Autodesk Inventor part; units mm, degrees
ref_plane "YZ Plane" through (0, 0, 0) normal (1, 0, 0) x (0, 1, 0)
ref_plane "XZ Plane" through (0, 0, 0) normal (0, 1, 0) x (-1, 0, 0)
ref_plane "XY Plane" through (0, 0, 0) normal (0, 0, 1) x (1, 0, 0)
sketch "Sketch1" plane through (0, 0, 0) normal (0, 0, 1) x (1, 0, 0)
  line L0 (0, 0) -> (20, 0)
  line L1 (20, 0) -> (20, -2.7984)
  line L2 (0, -2.7984) -> (0, 0)
  line L3 (0, 0) -> (20, 0)
  line L4 (20, 0) -> (20, -50)
  line L5 (20, -50) -> (0, -50)
  line L6 (0, -50) -> (0, 0)
  line L7 (0, 0) -> (5, 0)
  line L8 (0, -5) -> (0, 0)
  circle A0 centre (5, -5) radius 1.651
  line L9 (20, 0) -> (15, 0)
  line L10 (15, -5) -> (20, -5)
  line L11 (20, -5) -> (20, 0)
  circle A1 centre (15, -5) radius 1.651
  dimension "d1" = 20
  dimension "d2" = 50
  dimension "d6" = 5
  dimension "d7" = 5
  dimension "d9" = 3.302
extrude "Extrusion1" add sketch "Sketch1" along normal blind 5
sketch "Sketch2" plane through (0, 0, 5) normal (0, 0, 1) x (1, 0, 0)
  line L0 (20, 0) -> (0, 0)
  line L1 (10, 0) -> (5, 0)
  line L2 (5, 0) -> (5, 5)
  line L3 (5, 5) -> (10, 5)
  line L4 (10, 5) -> (10, 0)
  line L5 (10, 5) -> (2.5, 5)
  line L6 (2.5, 5) -> (2.5, 7.5)
  line L7 (2.5, 7.5) -> (10, 7.5)
  line L8 (10, 7.5) -> (10, 5)
  line L9 (2.5, 7.5) -> (17.5, 7.5)
  line L10 (17.5, 7.5) -> (17.5, 5)
  line L11 (17.5, 5) -> (2.5, 5)
  line L12 (2.5, 5) -> (2.5, 7.5)
  line L13 (10, 5) -> (15, 5)
  line L14 (15, 5) -> (15, 0)
  line L15 (15, 0) -> (10, 0)
  line L16 (10, 0) -> (10, 5)
  dimension "d12" = 5
  dimension "d13" = 5
  dimension "d14" = 7.5
  dimension "d15" = 2.5
  dimension "d16" = 15
  dimension "d17" = 2.5
  dimension "d18" = 5
  dimension "d19" = 5
extrude "Extrusion2" add sketch "Sketch2" against normal blind 5
sketch "Sketch3" plane through (0, 0, 0) normal (0, 0, -1) x (-1, 0, 0)
  line L0 (-5, 0) -> (-5, 5)
  line L1 (-5, 0) -> (-15, 0)
  line L2 (-15, 0) -> (-15, 5)
  line L3 (-15, 5) -> (-5, 5)
  line L4 (-5, 5) -> (-5, 0)
  point P0 (0, 0)
extrude "Extrusion3" cut sketch "Sketch3" against normal blind 1
sketch "Sketch4" plane through (0, 0, 0) normal (0, 0, -1) x (-1, 0, 0)
  line L0 (-5, 0) -> (0, 0)
  line L1 (-20, -50) -> (0, -50)
  line L2 (0, 0) -> (-20, 0)
  line L3 (-20, 0) -> (-20, -50)
  line L4 (-20, -50) -> (0, -50)
  line L5 (0, -50) -> (0, 0)
  line L6 (0, -50) -> (-5, -50)
  line L7 (-5, -50) -> (-5, -30)
  line L8 (-5, -30) -> (0, -30)
  line L9 (0, -30) -> (0, -50)
  line L10 (0, -50) -> (0, 0)
  line L11 (0, -50) -> (-5, -50)
  line L12 (-5, -50) -> (-5, -30)
  line L13 (-5, -30) -> (0, -30)
  line L14 (0, -30) -> (0, -50)
  line L15 (0, -50) -> (-20, -50)
  line L16 (-20, -50) -> (-20, -45)
  line L17 (-20, -45) -> (0, -45)
  line L18 (0, -45) -> (0, -50)
  dimension "d28" = 5
  dimension "d29" = 20
  dimension "d30" = 5
  dimension "d31" = 20
  dimension "d32" = 20
  dimension "d33" = 5
extrude "Extrusion4" add sketch "Sketch4" along normal blind 15 contours L17 L7 L1 L3 | L5 L1 L7 L17
sketch "Sketch5" plane through (0, 0, 5) normal (0, 0, 1) x (1, 0, 0)
  line L0 (20, -50) -> (20, 0)
  line L1 (20, 0) -> (0, 0)
  line L2 (0, 0) -> (0, -50)
  line L3 (0, -50) -> (20, -50)
  line L4 (20, -50) -> (20, 0)
  line L5 (10, -50) -> (15, -50)
  line L6 (15, -50) -> (15, -55)
  line L7 (15, -55) -> (10, -55)
  line L8 (10, -55) -> (10, -50)
  line L9 (15, -55) -> (5, -55)
  line L10 (5, -55) -> (5, -50)
  line L11 (5, -50) -> (15, -50)
  line L12 (15, -50) -> (15, -55)
  line L13 (10, -55) -> (17.5, -55)
  line L14 (17.5, -55) -> (17.5, -57.5)
  line L15 (17.5, -57.5) -> (10, -57.5)
  line L16 (10, -57.5) -> (10, -55)
  line L17 (17.5, -57.5) -> (2.5, -57.5)
  line L18 (2.5, -57.5) -> (2.5, -55)
  line L19 (2.5, -55) -> (17.5, -55)
  line L20 (17.5, -55) -> (17.5, -57.5)
  dimension "d36" = 5
  dimension "d37" = 5
  dimension "d38" = 10
  dimension "d39" = 5
  dimension "d40" = 7.5
  dimension "d41" = 2.5
  dimension "d42" = 15
  dimension "d43" = 2.5
extrude "Extrusion5" add sketch "Sketch5" against normal blind 5 contours L6 L7 L8 L3 | L8 L9 L10 L3 | L13 L14 L15 L16 L7 | L16 L17 L18 L19 L9
sketch "Sketch6" plane through (0, 0, 0) normal (0, 0, -1) x (-1, 0, 0)
  line L0 (-5, -55) -> (-5, -50)
  line L1 (-15, -50) -> (-5, -50)
  line L2 (-5, -55) -> (-15, -55)
  line L3 (-15, -55) -> (-15, -50)
  line L4 (-15, -50) -> (-5, -50)
  line L5 (-5, -50) -> (-5, -55)
  point P0 (0, 0)
extrude "Extrusion6" cut sketch "Sketch6" against normal blind 1
sketch "Sketch8" plane through (0, -45, 0) normal (0, 1, 0) x (1, 0, 0)
  line L0 (0, 15) -> (20, 15)
  line L1 (0, 15) -> (20, 15)
  line L2 (20, 15) -> (20, 0)
  line L3 (20, 0) -> (0, 0)
  line L4 (0, 0) -> (0, 15)
  line L5 (0, 0) -> (0, 15)
  line L6 (0, 7.5) -> (20, 7.5)
  line L7 (20, 0) -> (20, 15)
  line L8 (20, 0) -> (0, 15)
  line L9 (20, 15) -> (0, 0)
  line L10 (10, 7.5) -> (10, 15)
  line L11 (10, 7.5) -> (10, 0)
  line L12 (10, 7.5) -> (0, 0)
  line L13 (10, 7.5) -> (20, 0)
  line L14 (10, 7.5) -> (0, 15)
  line L15 (10, 7.5) -> (20, 15)
  circle A0 centre (5, 3.75) radius 1.651
  circle A1 centre (15, 3.75) radius 1.651
  circle A2 centre (15, 11.25) radius 1.651
  circle A3 centre (5, 11.25) radius 1.651
  dimension "d48" = 3.302
  dimension "d49" = 3.302
  dimension "d50" = 3.302
  dimension "d51" = 3.302
extrude "Extrusion7" cut sketch "Sketch8" against normal blind 5 contours A3 L8 | L8 A3 | A2 L9 | L9 A2 | A1 L8 | L8 A1 | A0 L9 | L9 A0
sketch "Sketch9" plane through (2.5, -57.5, 5) normal (0, -1, 0) x (1, 0, 0)
  line L0 (15, 0) -> (0, 0)
  line L1 (7.5, 0) -> (8, 0)
  line L2 (8, 0) -> (8, -0.5)
  line L3 (8, -0.5) -> (7.5, -0.5)
  line L4 (7.5, -0.5) -> (7.5, 0)
  line L5 (7.5, 0) -> (7, 0)
  line L6 (7, 0) -> (7, -0.5)
  line L7 (7, -0.5) -> (7.5, -0.5)
  line L8 (7.5, -0.5) -> (7.5, 0)
  point P0 (-2.5, -5)
  dimension "d54" = 0.5
  dimension "d55" = 0.5
  dimension "d56" = 0.5
  dimension "d57" = 0.5
extrude "Extrusion8" cut sketch "Sketch9" against normal blind 500
sketch "Sketch10" plane through (0, -45, 0) normal (0, 1, 0) x (1, 0, 0)
  circle A0 centre (5, 11.25) radius 1.651
  circle A1 centre (5, 11.25) radius 1.651
  circle A2 centre (5, 3.75) radius 1.651
  circle A3 centre (5, 3.75) radius 1.651
  circle A4 centre (15, 11.25) radius 1.651
  circle A5 centre (15, 11.25) radius 1.651
  circle A6 centre (15, 3.75) radius 1.651
  circle A7 centre (15, 3.75) radius 1.651
  circle A8 centre (5, 11.25) radius 3
  circle A9 centre (15, 11.25) radius 3
  circle A10 centre (5, 3.75) radius 3
  circle A11 centre (15, 3.75) radius 3
  line L0 (5, 14.25) -> (7.5981, 12.75)
  line L1 (7.5981, 12.75) -> (7.5981, 9.75)
  line L2 (7.5981, 9.75) -> (5, 8.25)
  line L3 (5, 8.25) -> (2.4019, 9.75)
  line L4 (2.4019, 9.75) -> (2.4019, 12.75)
  line L5 (2.4019, 12.75) -> (5, 14.25)
  line L6 (15, 14.25) -> (17.5981, 12.75)
  line L7 (17.5981, 12.75) -> (17.5981, 9.75)
  line L8 (17.5981, 9.75) -> (15, 8.25)
  line L9 (15, 8.25) -> (12.4019, 9.75)
  line L10 (12.4019, 9.75) -> (12.4019, 12.75)
  line L11 (12.4019, 12.75) -> (15, 14.25)
  line L12 (5, 6.75) -> (7.5981, 5.25)
  line L13 (7.5981, 5.25) -> (7.5981, 2.25)
  line L14 (7.5981, 2.25) -> (5, 0.75)
  line L15 (5, 0.75) -> (2.4019, 2.25)
  line L16 (2.4019, 2.25) -> (2.4019, 5.25)
  line L17 (2.4019, 5.25) -> (5, 6.75)
  line L18 (15, 6.75) -> (17.5981, 5.25)
  line L19 (17.5981, 5.25) -> (17.5981, 2.25)
  line L20 (17.5981, 2.25) -> (15, 0.75)
  line L21 (15, 0.75) -> (12.4019, 2.25)
  line L22 (12.4019, 2.25) -> (12.4019, 5.25)
  line L23 (12.4019, 5.25) -> (15, 6.75)
  point P0 (0, 0)
  dimension "d60" = 6
  dimension "d61" = 6
  dimension "d62" = 6
  dimension "d63" = 6
extrude "Extrusion9" cut sketch "Sketch10" against normal blind 2 contours L1 L2 L3 L4 L5 L0 | L7 L8 L9 L10 L11 L6 | L13 L14 L15 L16 L17 L12 | L19 L20 L21 L22 L23 L18
sketch "Sketch11" plane through (0, 0, 5) normal (0, 0, 1) x (1, 0, 0)
  circle A0 centre (5, -5) radius 1.651
  circle A1 centre (5, -5) radius 3
  circle A2 centre (15, -5) radius 1.651
  circle A3 centre (15, -5) radius 3
  line L0 (5, -2) -> (7.5981, -3.5)
  line L1 (7.5981, -3.5) -> (7.5981, -6.5)
  line L2 (7.5981, -6.5) -> (5, -8)
  line L3 (5, -8) -> (2.4019, -6.5)
  line L4 (2.4019, -6.5) -> (2.4019, -3.5)
  line L5 (2.4019, -3.5) -> (5, -2)
  line L6 (15, -2) -> (17.5981, -3.5)
  line L7 (17.5981, -3.5) -> (17.5981, -6.5)
  line L8 (17.5981, -6.5) -> (15, -8)
  line L9 (15, -8) -> (12.4019, -6.5)
  line L10 (12.4019, -6.5) -> (12.4019, -3.5)
  line L11 (12.4019, -3.5) -> (15, -2)
  point P0 (0, 0)
  dimension "d66" = 6
  dimension "d67" = 6
extrude "Extrusion10" cut sketch "Sketch11" against normal blind 2 contours L1 L2 L3 L4 L5 L0 | L7 L8 L9 L10 L11 L6
properties part number "Attachment"
The model under review builds one solid part; all positions refer to its coordinate system, in mm. A direction names the side the tool comes from. Round coordinates to 2 decimals unless told otherwise and drop trailing zeros. Write each loop counter-clockwise with the first axis right and the second up, starting at its lowest first coordinate (ties: lowest second). Pieces come first, ordered by that corner, then holes.
(1) We need section C-C on y = -21. Give the boundary of the cut face in (x, z), and give its area (3 significant figures).
(2) Insertion check: pin 1 (1.5 mm diameter, centred on y = -12, z = -1, fed in from -X); pin 2 (4 mm diameter, centred on x = 15, y = -4.5, fed in from +Z); pin 3 (5.5 mm diameter, centred on x = 4.5, z = -3.5, fed in from +Y); pin 4 (2 mm diameter, centred on x = 11, y = -8.5, fed in from -Z). Each pin has a flat end and moves straight along its axis. Give the tip position at first contact, or say it passes through.
(3) Machinability: for faces 4 (the flat face through (11.8, 5, 0.3)), 5 (the flat face through (16.3, -46, -13.5)), 6 (the flat face through (16.32, -7.24, 4.01)), 7 (the flat face through (10, 6, 0)), 8 (the flat face through (10, -56, 0)), which of the approach directions +Z, -Z, +X, -X, +Y, -Y give a long, thin tool a straight path to every point of the face, cutting with its end or side? Answer none if there is none.
(4) Wall thickness on L1, parallel to Z at x = 5, y = -48.5; L2, parallel to X at y = -49, z = -3.75; L3, parallel to Z at x = 6.5, y = -47.5: over which ranges is each line inside the solid? List them lowest first.
(5) We need section A-A on y = -5. Give the boundary of the cut face in (x, z).
(6) We need section D-D on x = 14. Give the number of separate pieces and of enclosed holes in the cut face, and give its area (3 significant figures).
(7) We need section B-B on z = -11.25. Give the boundary of the cut face in (x, y), and give its area (3 significant figures).
(8) Mouldability with a two-part tool opening along X and no side actions: class faces 1 (the flat face through (15, -52, 3)), 2 (the flat face through (10, -45, -7)), 3 (the flat face through (3.7, -46, -6)) as +X half, -X half, draft (parallel to the pull), parting line (faces both ways), or undercut.
Findings below:
1. outline: (0, 0) - (20, 0) - (20, 5) - (10.5, 5) - (10.5, 4.5) - (9.5, 4.5) - (9.5, 5) - (0, 5) - close
1. area: 99.5 mm2
2. pin 1: passes through
2. pin 2: stops at z = 3
2. pin 3: stops at y = -45
2. pin 4: stops at z = 0
3. face 4: -Z
3. face 5: +Y
3. face 6: +Z
3. face 7: -Z, +X, -X, +Y
3. face 8: -Z, +X, -X, -Y
4. L1: z = -15 to -12.9, -9.6 to -5.4, -2.1 to 5
4. L2: x = 0 to 3.35, 6.65 to 13.35, 16.65 to 20
4. L3: z = -15 to -11.94, -10.56 to -4.44, -3.06 to 5
5. outline: (0, 0) - (3.35, 0) - (3.35, 3) - (2.4, 3) - (2.4, 5) - (0, 5) - close; (6.65, 0) - (13.35, 0) - (13.35, 3) - (12.4, 3) - (12.4, 5) - (10.5, 5) - (10.5, 4.5) - (9.5, 4.5) - (9.5, 5) - (7.6, 5) - (7.6, 3) - (6.65, 3) - close; (16.65, 0) - (20, 0) - (20, 5) - (17.6, 5) - (17.6, 3) - (16.65, 3) - close
6. separate pieces: 4
6. enclosed holes: 0
6. area: 337 mm2
7. outline: (0, -50) - (3.35, -50) - (3.35, -47) - (2.4, -47) - (2.4, -45) - (0, -45) - close; (6.65, -50) - (13.35, -50) - (13.35, -47) - (12.4, -47) - (12.4, -45) - (7.6, -45) - (7.6, -47) - (6.65, -47) - close; (16.65, -50) - (20, -50) - (20, -45) - (17.6, -45) - (17.6, -47) - (16.65, -47) - close
7. area: 59.4 mm2
8. face 1: +X half
8. face 2: draft
8. face 3: undercut
